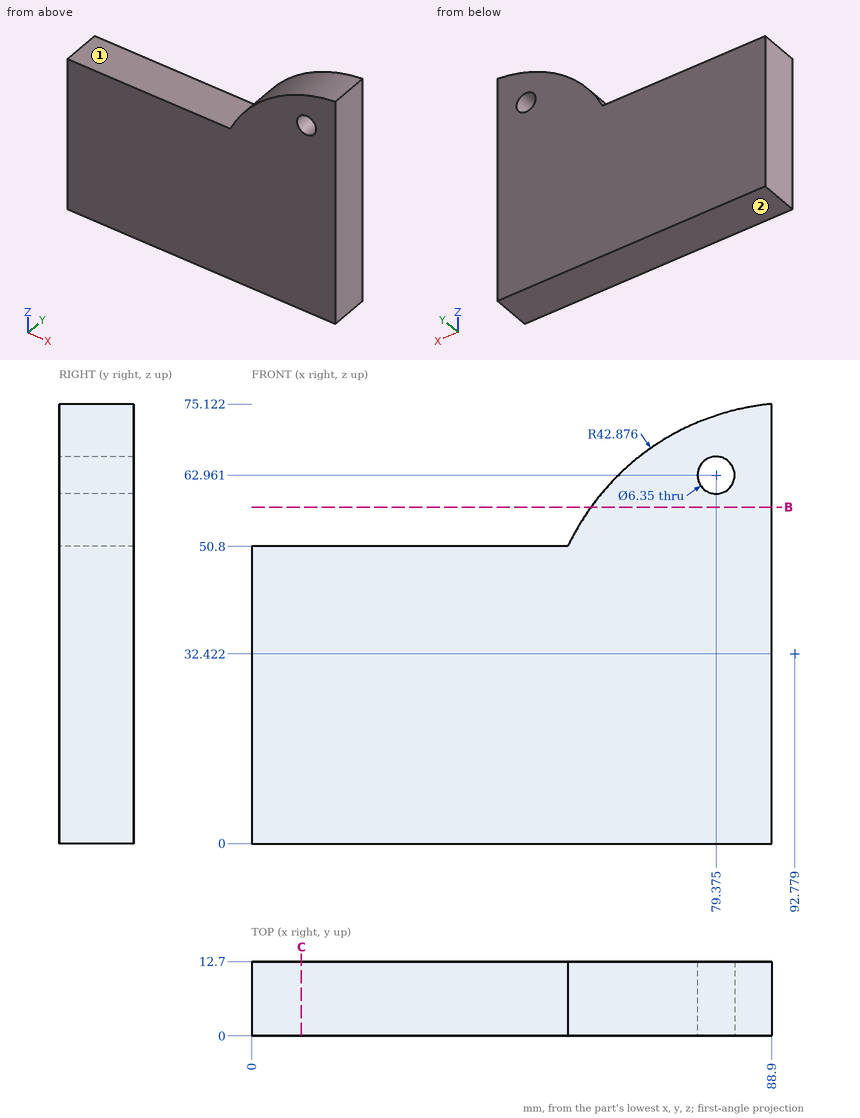
Input: dimensioned drawing with shaded views. Units: mm. Origin: part minimum x, y, z. A direction names the side the tool comes from. Round coordinates to 2 decimals unless told otherwise and drop trailing zeros. Order: outer loops, then holes, each group sorted by start corner. A loop starts at its lowest first (then second) coordinate and runs counter-clockwise, first axis right, second up. Notation, with made-up numbers: (58.25, 54.25) -> (80.25, 54.25) arc R24 ccw to (80.25, 82.25) -> close; hole circle Ø8 at (18, 2). An arc over 180 degrees is marked (long way). One line per item, written item: value. Start each with the question number.
Q1. Section query B-B (z = 57.5). Return the cut outline in (x, y).
Q2. Access query for the marked faces 1 and 2. Directions: +Z, -Z, +X, -X, +Y, -Y. A direction counts if a zero-diameter tool reaches every point of the face in a straight line with its end or side. Return the directions, or none.
Q3. Section query C-C (x = 8.5). Return the cut outline in (y, z), plus the area to 3 significant figures.
Q4. Material intervals for probe 1 along Z at (x, y) = (29, 5); probe 2 along X at (y, z) = (11.75, 71.5) (1 decimal); probe 3 along Z at (x, y) = (83, 8.5), sorted ascending.
Findings below:
1. outline: (58, 0) -> (88.9, 0) -> (88.9, 12.7) -> (58, 12.7) -> close
2. face 1: +Z, -X, +Y, -Y
2. face 2: -Z, +X, -X, +Y, -Y
3. outline: (0, 0) -> (12.7, 0) -> (12.7, 50.8) -> (0, 50.8) -> close
3. area: 645 mm²
4. probe 1: 0 to 50.8
4. probe 2: 75.1 to 88.9
4. probe 3: 0 to 74.17
